Here's how the part is built. I have some questions about the finished solid (model axes, mm). A direction names the side the tool comes from. Give positions to 0.01 mm unless a question says otherwise; leave off trailing zeros. Order: outer loops, then holes, each group sorted by start corner. A loop starts at its lowest first (then second) coordinate and runs counter-clockwise, first axis right, second up. Notation, with made-up numbers: M 19.5,-28 L 29.5,-28 A13 ccw 29.5,-11 Z; hole C -6,-39.5 d1. An arc over 180 degrees is marked long. One line per item, written item: value. Start each with the question number.
from build123d import *

# Parameters (mm, degrees)
BOSS_EXTRUDE1_DEPTH = 73.5
BOSS_EXTRUDE2_DEPTH = 36.75


with BuildPart() as part:
    # Sketch2 → Boss-Extrude1 (new, symmetric)
    with BuildSketch(Plane(origin=(0, 0, 0), x_dir=(1, 0, 0), z_dir=(0, 1, 0))):
        Polygon((24.192265263, 0), (14.646810718, 28), (-14.646810718, 28), (-24.192265263, 0), align=None)
        Polygon((12.678900893, 25.25), (-12.678900893, 25.25), (-20.349355439, 2.75), (20.349355439, 2.75), align=None, mode=Mode.SUBTRACT)
    extrude(amount=BOSS_EXTRUDE1_DEPTH, both=True)

    # Sketch3 → Boss-Extrude2 (add, symmetric)
    # profile 1 of 2: a face of its own
    with BuildSketch(Plane(origin=(0, 0, 0), x_dir=(1, 0, 0), z_dir=(0, 1, 0))):
        Polygon((-23.169537991, 3), (-48.169537991, 3), (-55.669537991, 25), (-15.669537991, 25), (-14.646810718, 28), (-85.985886699, 28), (-95.531341245, 0), (-24.192265263, 0), align=None)
        Polygon((-58.660175088, 25.25), (-50.989720543, 2.75), (-91.68843142, 2.75), (-84.017976875, 25.25), align=None, mode=Mode.SUBTRACT)
    # profile 2 of 2: a face of its own
    with BuildSketch(Plane(origin=(0, 0, 0), x_dir=(1, 0, 0), z_dir=(0, 1, 0))):
        Polygon((24.192265263, 0), (23.169537991, 3), (48.169537991, 3), (55.669537991, 25), (15.669537991, 25), (14.646810718, 28), (85.985886699, 28), (95.531341245, 0), align=None)
        Polygon((84.017976875, 25.25), (58.660175088, 25.25), (50.989720543, 2.75), (91.68843142, 2.75), align=None, mode=Mode.SUBTRACT)
    extrude(amount=BOSS_EXTRUDE2_DEPTH, both=True)


solid = part.part
Item 1: I want a section at D-D on y = 29. Write out the boundary of the cut face in (x, z).
Item 2: We'd pull the mould along Z, two halves only. Please class faces 3 (the face through (-51.87, -0.51, -13.85)), 4 (the face through (1, 1, -28)), 5 (the face through (35, 1, -3)), 6 (the face through (-1, 1, 0)): +Z half, -Z half, draft (parallel to the pull), parting line (faces both ways), or undercut.
Item 3: Please list where these lines run through material, in increasing order: probe 1 along Z at (x, y) = (32.5, -33.5); probe 2 along Z at (x, y) = (-59.5, -9.5); probe 3 along X at (y, z) = (34.5, -21.5). Write a range as [from, to].
Item 4: For faces 1 (the face through (71, 1, -2.75)), 2 (the face through (0, 73.5, -2)), which set-ups out of +Z, -Z, +X, -X, +Y, -Y let a thin tool reach every point of the face, with its end or its side?
Item 5: I want a section at A-A on x = -45. Write out the boundary of the cut face in (y, z).
Item 6: Will these pins go through, and if not, where does the flat tip stop? P1, Ø8, axis at x = 21.5, y = -7, coming from the +Z side; P2, Ø1.5, axis at y = -35.5, z = -16, coming from the +X side; P3, Ø8.5, axis at x = 58, z = -13.5, coming from the +Y side; P4, Ø5, axis at y = 49, z = -16.5, coming from the -X side.
Item 7: I want a section at B-B on y = 45. Write out the boundary of the cut face in (x, z).
Item 8: I want a section at C-C on z = -18. Write out the boundary of the cut face in (x, y), plus the area to 3 significant figures.
Answer below:
1. outline: M -95.53,0 L -85.99,-28 L 85.99,-28 L 95.53,0 Z; hole M -91.69,-2.75 L -84.02,-25.25 L -58.66,-25.25 L -50.99,-2.75 Z; hole M -55.67,-25 L -15.67,-25 L -23.17,-3 L -48.17,-3 Z; hole M -20.35,-2.75 L -12.68,-25.25 L 12.68,-25.25 L 20.35,-2.75 Z; hole M 15.67,-25 L 55.67,-25 L 48.17,-3 L 23.17,-3 Z; hole M 50.99,-2.75 L 58.66,-25.25 L 84.02,-25.25 L 91.69,-2.75 Z
2. face 3: undercut
2. face 4: -Z half
2. face 5: undercut
2. face 6: +Z half
3. probe 1: z = [-28, -25], [-3, 0]
3. probe 2: z = [-28, -25.25], [-2.75, 0]
3. probe 3: x = [-88.2, -85.3], [-57.38, -54.48], [-16.86, -13.96], [13.96, 16.86], [54.48, 57.38], [85.3, 88.2]
4. face 1: +Y, -Y
4. face 2: +Z, -Z, +X, -X, +Y
5. outline: M -36.75,-28 L 36.75,-28 L 36.75,-25 L -36.75,-25 Z; M -36.75,-3 L 36.75,-3 L 36.75,0 L -36.75,0 Z
6. P1: stops at z = 0
6. P2: stops at x = 90.33
6. P3: stops at y = 36.75
6. P4: stops at x = -19.42
7. outline: M -24.19,0 L -14.65,-28 L 14.65,-28 L 24.19,0 Z; hole M -20.35,-2.75 L -12.68,-25.25 L 12.68,-25.25 L 20.35,-2.75 Z
8. outline: M -89.39,-36.75 L -86.49,-36.75 L -86.49,36.75 L -89.39,36.75 Z; M -56.19,-36.75 L -53.28,-36.75 L -53.28,36.75 L -56.19,36.75 Z; M -18.06,-73.5 L -15.15,-73.5 L -15.15,73.5 L -18.06,73.5 Z; M 15.15,-73.5 L 18.06,-73.5 L 18.06,73.5 L 15.15,73.5 Z; M 53.28,-36.75 L 56.19,-36.75 L 56.19,36.75 L 53.28,36.75 Z; M 86.49,-36.75 L 89.39,-36.75 L 89.39,36.75 L 86.49,36.75 Z
8. area: 1,710 mm²
